```python
from build123d import *

# Parameters (mm, degrees)
SKETCH1_W           = 43.6
SKETCH1_H           = 95
BOSS_EXTRUDE1_DEPTH = 10
SKETCH2_R           = 3.9
BOSS_EXTRUDE2_DEPTH = 4
SKETCH5_R           = 20
SKETCH5_R_2         = 19
BOSS_EXTRUDE4_DEPTH = 10
SKETCH6_W           = 15
SKETCH6_H           = 43.6
CUT_EXTRUDE1_DEPTH  = 10
FILLET1_R           = 20
CUT_EXTRUDE2_START  = -3
SKETCH7_R           = 19
CUT_EXTRUDE2_DEPTH  = 3


with BuildPart() as part:
    # Sketch1 → Boss-Extrude1 (new body)
    with BuildSketch(Plane(origin=(0, 0, 0), x_dir=(0, 1, 0), z_dir=(0, 0, 1))):
        Rectangle(SKETCH1_W, SKETCH1_H)
    extrude(amount=BOSS_EXTRUDE1_DEPTH)

    # Sketch2 → Boss-Extrude2 (add)
    with BuildSketch(Plane(origin=(0, 0, 0), x_dir=(1, 0, 0), z_dir=(0, 0, -1))):
        with Locations(Location((0, 12.45, 0), (0, 0, 180))):
            Circle(SKETCH2_R)
        with Locations(Location((0, -12.45, 0), (0, 0, 180))):
            Circle(SKETCH2_R)
    extrude(amount=BOSS_EXTRUDE2_DEPTH)

    # Sketch5 → Boss-Extrude4 (add)
    # profile 1 of 2: a face of its own
    with BuildSketch(Plane.XY.offset(10)):
        with Locations((-25.5, 0)):
            Circle(SKETCH5_R)
        with Locations((-25.5, 0)):
            Circle(SKETCH5_R_2, mode=Mode.SUBTRACT)
    # profile 2 of 2: a face of its own
    with BuildSketch(Plane.XY.offset(10)):
        with Locations((25.5, 0)):
            Circle(SKETCH5_R)
        with Locations((25.5, 0)):
            Circle(SKETCH5_R_2, mode=Mode.SUBTRACT)
    extrude(amount=BOSS_EXTRUDE4_DEPTH)

    # Sketch6 → Cut-Extrude1 (cut)
    with BuildSketch(Plane.XY.offset(20)):
        with Locations((-25.5, 0)):
            Rectangle(SKETCH6_W, SKETCH6_H)
        with Locations((25.5, 0)):
            Rectangle(SKETCH6_W, SKETCH6_H)
    extrude(amount=-CUT_EXTRUDE1_DEPTH, mode=Mode.SUBTRACT)

    # Fillet1
    fillet1_edges = [part.edges().sort_by_distance(p)[0] for p in [
        (47.5, 21.8, 5),
        (47.5, -21.8, 5),
        (-47.5, -21.8, 5),
        (-47.5, 21.8, 5),
    ]]
    fillet(fillet1_edges, radius=FILLET1_R)

    # Sketch7 → Cut-Extrude2 (cut)
    with BuildSketch(Plane.XY.offset(10).offset(CUT_EXTRUDE2_START)):
        with Locations(Location((-25.5, 0, 0), (0, 0, 246.750437409))):
            Circle(SKETCH7_R)
        with Locations(Location((25.5, 0, 0), (0, 0, 180))):
            Circle(SKETCH7_R)
    extrude(amount=CUT_EXTRUDE2_DEPTH, mode=Mode.SUBTRACT)


solid = part.part
```
The model under review builds one solid part; all positions refer to its coordinate system, in mm. A direction names the side the tool comes from. Round coordinates to 2 decimals unless told otherwise and drop trailing zeros. Write each loop counter-clockwise with the first axis right and the second up, starting at its lowest first coordinate (ties: lowest second). Pieces come first, ordered by that corner, then holes. Notation, with made-up numbers: (-1, -28.5) - (55, -28.5) arc R10 cw to (55, -18.5) - close; hole circle Ø11 at (74, 18.5). An arc over 180 degrees is marked (long way). Answer as CSV lines item,"result". Start each with the question number.
(1) For pin 1 Ø12 at (x, z) = (13.5, 17) entering from -Y; pin 2 Ø11.5 at (x, y) = (-31.5, 1) entering from +Z; pin 3 Ø1.5 at (y, z) = (-14.5, 12.5) entering from +X, all flat-tipped, find the tip position at first contact; note any pin that passes through.
(2) We need section A-A on z = 17.75. State the section outline as (x, y) points.
(3) We need section D-D on z = -1. State the section outline as (x, y) points, plus the area to 3 significant figures.
(4) To check wall thickness, follow line 1 (X direction, y = -6.5, z = 9); line 2 (X direction, y = 8, z = 7.25); line 3 (Z direction, x = -4.5, y = -8). State the ranges of each line that lie inside material, in increasing order.
(5) We need section C-C on y = -4.5. State the section outline as (x, z) points.
(6) We need section B-B on x = 25.5. State the section outline as (y, z) points.
(7) For faces 4 (the cylindrical face through (0.845, -16.257, -1.972)), 5 (the flat face through (-47.5, 0, 5)), 6 (the cylindrical face through (-45.497, 0.332, 14.93)), 7 (the cylindrical face through (45.497, -0.332, 14.93)), 8 (the cylindrical face through (-5.503, -0.332, 14.93)), list the 3-axis set-ups (+Z, -Z, +X, -X, +Y, -Y) from which the entire face can be reached by the end or side of a thin tool; tool diameter is ignored.
(8) Draft analysis for pull direction Y (two halves, no side actions). For faces 1 (the flat face through (0, 0, 10)), 2 (the cylindrical face through (5.503, 0.332, 14.93)), 3 (the flat face through (-25, 0, 7)), state which applies: pulls with the +Y half, pulls with the -Y half, needs draft (parallel to the pull), parting line crosses it, or undercut.
Worked answers:
1,pin 1,"y = -18.54"
1,pin 2,"z = 7"
1,pin 3,"x = 40.02"
2,outline,"(-33, -18.54) - (-33, -17.46) arc R19 cw to (-33, 17.46) - (-33, 18.54) arc R20 ccw to start; (-18, -18.54) arc R20 ccw to (-18, 18.54) - (-18, 17.46) arc R19 cw to (-18, -17.46) - close; (18, -18.54) - (18, -17.46) arc R19 cw to (18, 17.46) - (18, 18.54) arc R20 ccw to start; (33, -18.54) arc R20 ccw to (33, 18.54) - (33, 17.46) arc R19 cw to (33, -17.46) - close"
3,outline,"circle Ø7.8 at (0, -12.45); circle Ø7.8 at (0, 12.45)"
3,area,"95.6 mm²"
4,line 1,"-46.94 to -43.35, -7.65 to 7.65, 43.35 to 46.94"
4,line 2,"-46.51 to -42.73, -8.27 to 8.27, 42.73 to 46.51"
4,line 3,"0 to 10"
5,outline,"(-47.32, 0) - (47.32, 0) - (47.32, 10) - (44.99, 10) - (44.99, 20) - (43.96, 20) - (43.96, 7) - (7.04, 7) - (7.04, 20) - (6.01, 20) - (6.01, 10) - (-6.01, 10) - (-6.01, 20) - (-7.04, 20) - (-7.04, 7) - (-43.96, 7) - (-43.96, 20) - (-44.99, 20) - (-44.99, 10) - (-47.32, 10) - close"
6,outline,"(-21.8, 0) - (21.8, 0) - (21.8, 10) - (19, 10) - (19, 7) - (-19, 7) - (-19, 10) - (-21.8, 10) - close"
7,face 4,"-Z"
7,face 5,"+Z, -Z, -X, +Y, -Y"
7,face 6,"+Z, -X"
7,face 7,"+Z, +X"
7,face 8,"+Z"
8,face 1,"needs draft"
8,face 2,"parting line crosses it"
8,face 3,"undercut"
